```python
from build123d import *

# Parameters (mm, degrees)
SKETCH1_W               = 44.958
SKETCH1_H               = 44.958
BOSS_EXTRUDE1_DEPTH     = 298.45
SKETCH2_R               = 9.525
BOSS_EXTRUDE2_DEPTH     = 38.1
CUT_EXTRUDE1_DEPTH      = 341.282867193
CUT_EXTRUDE1_DEPTH_BACK = 341.282867193
CUT_EXTRUDE2_DEPTH      = 341.282867193
CUT_EXTRUDE2_DEPTH_BACK = 341.282867193
SKETCH4_R               = 3.175
SKETCH5_W               = 5
SKETCH5_H               = 20
CUT_EXTRUDE3_DEPTH      = 32
SKETCH6_R               = 3.175
BOSS_EXTRUDE3_DEPTH     = 9.525
SKETCH7_W               = 6
SKETCH7_H               = 44.958
CUT_EXTRUDE4_DEPTH      = 19.05
FILLET1_R               = 2


with BuildPart() as part:
    # Sketch1 → Boss-Extrude1 (new body)
    with BuildSketch(Plane(origin=(0, 0, 0), x_dir=(1, 0, 0), z_dir=(0, 1, 0))):
        Rectangle(SKETCH1_W, SKETCH1_H)
    extrude(amount=BOSS_EXTRUDE1_DEPTH)

    # Sketch2 → Boss-Extrude2 (add)
    with BuildSketch(Plane(origin=(0, 298.45, 0), x_dir=(1, 0, 0), z_dir=(0, 1, 0))):
        with Locations(Location((0, -7.239, 0), (0, 0, 90))):
            Circle(SKETCH2_R)
    extrude(amount=BOSS_EXTRUDE2_DEPTH)

    # Sketch3 → Cut-Extrude1 (cut, two sides: drawn at the far end of the back side and taken through both)
    with BuildSketch(Plane.ZY.offset(22.479).offset(-CUT_EXTRUDE1_DEPTH_BACK)):
        with BuildLine():
            Line((-2.286, 327.025), (-2.286, 352.425))
            Line((-2.286, 352.425), (16.764, 352.425))
            Line((16.764, 352.425), (16.764, 327.025))
            ThreePointArc((16.764, 327.025), (7.239, 336.55), (-2.286, 327.025))
        make_face()
    extrude(amount=CUT_EXTRUDE1_DEPTH + CUT_EXTRUDE1_DEPTH_BACK, mode=Mode.SUBTRACT)

    # Sketch4 → Cut-Extrude2 (cut, two sides: drawn at the far end of the back side and taken through both)
    with BuildSketch(Plane.ZY.offset(22.479).offset(-CUT_EXTRUDE2_DEPTH_BACK)):
        with Locations((7.239, 329.946)):
            Circle(SKETCH4_R)
    extrude(amount=CUT_EXTRUDE2_DEPTH + CUT_EXTRUDE2_DEPTH_BACK, mode=Mode.SUBTRACT)

    # Sketch5 → Cut-Extrude3 (cut)
    with BuildSketch(Plane(origin=(0, 348.45, 0), x_dir=(1, 0, 0), z_dir=(0, 1, 0))):
        with Locations((0, -7.239)):
            Rectangle(SKETCH5_W, SKETCH5_H)
    extrude(amount=-CUT_EXTRUDE3_DEPTH, mode=Mode.SUBTRACT)

    # Sketch6 → Boss-Extrude3 (add, symmetric)
    with BuildSketch(Plane(origin=(0, 0, 0), x_dir=(0, 0, -1), z_dir=(1, 0, 0))):
        with BuildLine():
            Line((2.114129326, 0), (-16.592129326, 0))
            Line((-16.592129326, 0), (-12.967366216, -9.958954794))
            ThreePointArc((-12.967366216, -9.958954794), (-7.239, -13.97), (-1.510633784, -9.958954794))
            Line((-1.510633784, -9.958954794), (2.114129326, 0))
        make_face()
        with Locations(Location((-7.239, -7.874, 0), (0, 0, 180))):
            Circle(SKETCH6_R, mode=Mode.SUBTRACT)
    extrude(amount=BOSS_EXTRUDE3_DEPTH, both=True)

    # Sketch7 → Cut-Extrude4 (cut)
    with BuildSketch(Plane.XZ):
        Rectangle(SKETCH7_W, SKETCH7_H)
    extrude(amount=CUT_EXTRUDE4_DEPTH, mode=Mode.SUBTRACT)

    # Fillet1
    fillet1_edges = [part.edges().sort_by_distance(p)[0] for p in [
        (-22.479, 298.45, 0),
        (0, 298.45, 22.479),
        (22.479, 298.45, 0),
        (0, 0, 22.479),
        (-22.479, 0, 0),
        (0, 0, -22.479),
        (22.479, 0, 0),
        (0, 298.45, -22.479),
        (22.479, 149.225, 22.479),
        (-22.479, 149.225, 22.479),
        (-22.479, 149.225, -22.479),
        (22.479, 149.225, -22.479),
    ]]
    fillet(fillet1_edges, radius=FILLET1_R)


solid = part.part
```
The listing builds one solid part. Answer for the finished solid, in the listing's coordinates (mm). A direction names the side the tool comes from. Give positions to 0.01 mm unless a question says otherwise; leave off trailing zeros. Order: outer loops, then holes, each group sorted by start corner. A loop starts at its lowest first (then second) coordinate and runs counter-clockwise, first axis right, second up.
Item 1: Find the intervals of material crossed by probe 1 along Y at (x, z) = (-10, -16.5); probe 2 along X at (y, z) = (310, 8); probe 3 along Y at (x, z) = (2, 5.5), in increasing order.
From the geometry:
probe 1: y = 0 to 298.45
probe 2: x = -9.49 to 9.49
probe 3: y = 0 to 316.45
Item 2: The part is cut by section B-B, the plane y = 308.5. Give the vertices of the cut face in (x, z) (3 decimals), and give its area (3 significant figures).
From the geometry:
outline: circle Ø19.05 at (0, 7.239)
area: 285 mm2
Item 3: Given pin 1 Ø9 at (y, z) = (327.5, 5.5) entering from +X (3 decimals); pin 2 Ø1 at (x, z) = (12.5, -9) entering from +Y; pin 3 Ø20 at (y, z) = (330, 6.5) entering from -X (3 decimals), each flat-ended and moving along its own axis, determine where each tip first touches the part or whether it passes through.
From the geometry:
pin 1: stops at x = 9.525
pin 2: stops at y = 298.45
pin 3: stops at x = -9.525
Item 4: Which of the six approach directions +Z, -Z, +X, -X, +Y, -Y give full straight-line access (tool end or side, diameter ignored) to faces 1 (the face through (9.525, -4, 7)), 2 (the face through (-9.525, -4, 7)), 3 (the face through (2.5, 324, 7)), 4 (the face through (3.65, 313, -1.56))?
From the geometry:
face 1: +Z, -Z, +X, -Y
face 2: +Z, -Z, -X, -Y
face 3: +Z, -Z, +Y
face 4: +Y
Item 5: The part is cut by section A-A, the plane z = -16. Give the vertices of the cut face in (x, y).
From the geometry:
outline: (-22.48, 2) arc R2 ccw to (-20.48, 0) - (20.48, 0) arc R2 ccw to (22.48, 2) - (22.48, 296.45) arc R2 ccw to (20.48, 298.45) - (-20.48, 298.45) arc R2 ccw to (-22.48, 296.45) - close
Item 6: For a pull along X with two mould halves and no side action, classify faces 5 (the face through (22.479, 147, 0)), 6 (the face through (3, -4, 7)), 7 (the face through (-6.22, -13.97, 7.34)) as pulls with the +X half, pulls with the -X half, needs draft (parallel to the pull), parting line crosses it, or undercut.
From the geometry:
face 5: pulls with the +X half
face 6: undercut
face 7: needs draft
